Job drawing, mm, ordinate dimensions from the low corner. One solid piece. Give positions to 0.01 mm unless a question says otherwise; leave off trailing zeros. Order: outer loops, then holes, each group sorted by start corner. A loop starts at its lowest first (then second) coordinate and runs counter-clockwise, first axis right, second up. Notation, with made-up numbers: (-6.5, 32.25) - (42.5, 32.25) arc R24 cw to (42.5, 48.25) - close; hole circle Ø4 at (31.5, 58.5). An arc over 180 degrees is marked (long way). Use a Markdown table: item, result. Add a question column.
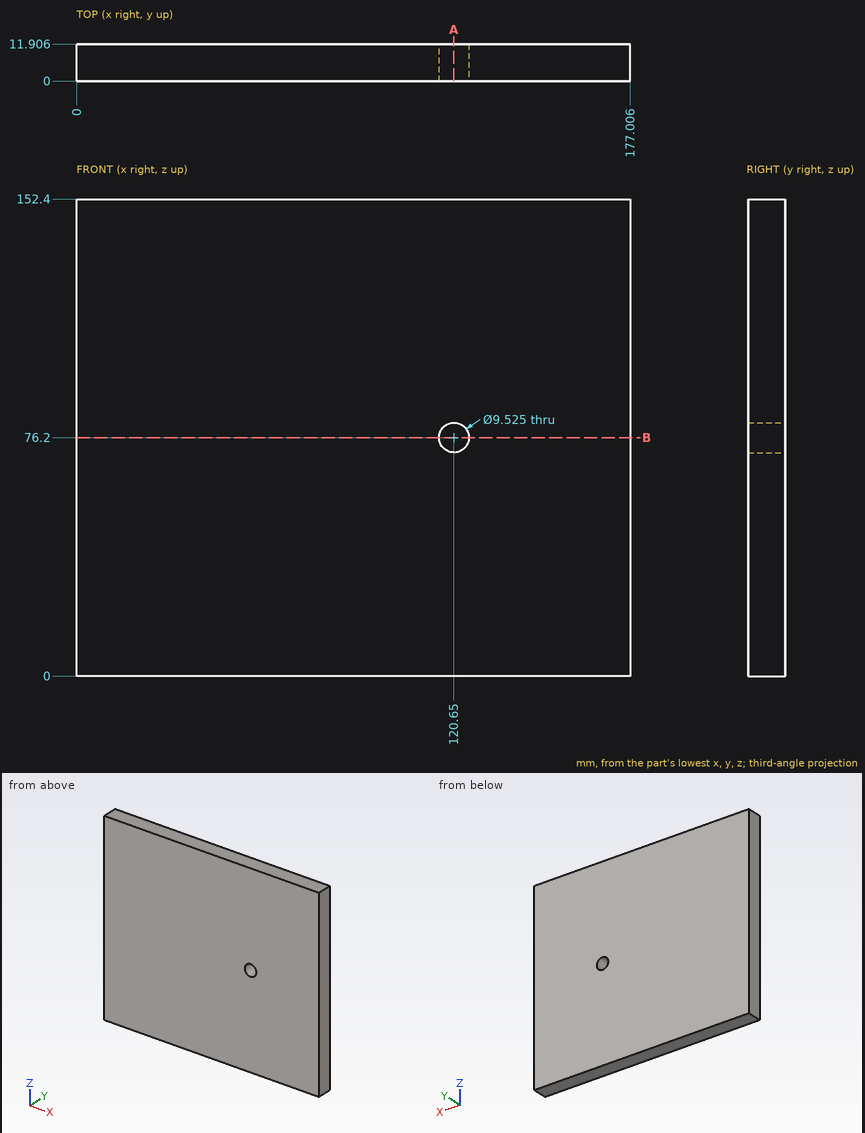
1. Cut at A-A (x = 120.65). Write the cut outline in (y, z).
2. Drill centre lines: probe 1 along Z at (x, y) = (120.65, 8.5); probe 2 along X at (y, z) = (7, 76.2); probe 3 along Z at (x, y) = (117, 5.25). Where is each one in solid material? Low to high. Write a range as [from, to].
3. Cut at B-B (z = 76.2). Write the cut outline in (x, y), plus the area to 3 significant figures.
Responses:
| question | item | result |
|---|---|---|
| 1 | outline | (0, 0) - (11.91, 0) - (11.91, 71.44) - (0, 71.44) - close; (0, 80.96) - (11.91, 80.96) - (11.91, 152.4) - (0, 152.4) - close |
| 2 | probe 1 | z = [0, 71.44], [80.96, 152.4] |
| 2 | probe 2 | x = [0, 115.89], [125.41, 177.01] |
| 2 | probe 3 | z = [0, 73.14], [79.26, 152.4] |
| 3 | outline | (0, 0) - (115.89, 0) - (115.89, 11.91) - (0, 11.91) - close; (125.41, 0) - (177.01, 0) - (177.01, 11.91) - (125.41, 11.91) - close |
| 3 | area | 1,990 mm² |
